Source: CAD feature listing. Evaluate the final solid. Frame: model axes, mm. Face numbers are marked on the shaded views. A direction names the side the tool comes from. Give positions to 0.01 mm unless a question says otherwise; leave off trailing zeros. Loops run counter-clockwise (first coordinate to the right, second up) from the corner with the lowest first, then second, coordinate; pieces in that order, holes last. Notation, with made-up numbers: M -31,79 L -15,79 A29 ccw -15,112 Z; hole C 41.5,0 d2. An arc over 180 degrees is marked long. Answer in a Markdown table with one row per item.
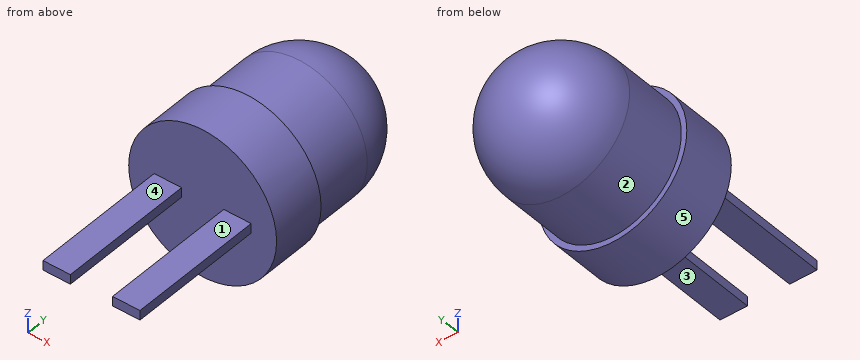
```python
from build123d import *

# Parameters (mm, degrees)
SKETCH2_W                = 1
SKETCH2_H                = 0.35
BOSS_EXTRUDE1_DEPTH      = 5
BOSS_EXTRUDE1_DEPTH_BACK = 5


with BuildPart() as part:
    # Sketch1 → Revolve1 (revolve)
    with BuildSketch(Plane.XY):
        with BuildLine():
            Line((0, 0), (0, 6.825))
            ThreePointArc((0, 6.825), (1.767766953, 6.092766953), (2.5, 4.325))
            Line((2.5, 4.325), (2.5, 2))
            Line((2.5, 2), (2.7, 2))
            Line((2.7, 2), (2.7, 0))
            Line((2.7, 0), (0, 0))
        make_face()
    revolve(axis=Axis((0, 0, 0), (0, 1, 0)))

    # Sketch2 → Boss-Extrude1 (add, two sides)
    with BuildSketch(Plane.XZ) as boss_extrude1_sk:
        with Locations((1.27, 0)):
            Rectangle(SKETCH2_W, SKETCH2_H)
        with Locations((-1.27, 0)):
            Rectangle(SKETCH2_W, SKETCH2_H)
    extrude(amount=BOSS_EXTRUDE1_DEPTH)
    extrude(boss_extrude1_sk.sketch, amount=-BOSS_EXTRUDE1_DEPTH_BACK)


solid = part.part
```
1) Pin query (flat end, axial travel): pin 1 Ø1.1 at (x, y) = (1, -3) entering from -Z (3 decimals); pin 2 Ø1.5 at (y, z) = (2.5, 0) entering from -X; pin 3 Ø1 at (x, y) = (1.5, 0) entering from -Z. Return the tip coordinate at first contact, or that it passes through.
Reply:
| item | result |
|---|---|
| pin 1 | stops at z = -0.175 |
| pin 2 | stops at x = -2.7 |
| pin 3 | stops at z = -2.51 |
2) Material intervals for L1, parallel to Y at x = -2.4, z = -1.1; L2, parallel to Z at x = 1.8, y = 2.75; L3, parallel to X at y = 2.75, z = -1.05, sorted ascending.
Reply:
| item | result |
|---|---|
| L1 | y = 0 to 2 |
| L2 | z = -1.73 to 1.73 |
| L3 | x = -2.27 to 2.27 |
3) Section C-C, the plane x = 0. Return loops of the section in (y, z) (3 decimals).
Reply:
| item | result |
|---|---|
| outline | M 0,-2.7 L 2,-2.7 L 2,-2.5 L 4.325,-2.5 A2.5 ccw 4.325,2.5 L 2,2.5 L 2,2.7 L 0,2.7 Z |
4) Section D-D, the plane y = 2.75. Return loops of the section in (x, z), then the cut area to 3 significant figures.
Reply:
| item | result |
|---|---|
| outline | C 0,0 d5 |
| area | 19.6 mm² |
5) Pull-direction query (X, two-part tool) for the marked faces 4 and 5; classes: released by +X, released by -X, zero draft, split by the parting line, or undercut.
Reply:
| item | result |
|---|---|
| face 4 | zero draft |
| face 5 | split by the parting line |
6) Set-up query: the marked faces 1, 2 and 3. Return all of +Z, -Z, +X, -X, +Y, -Y with unobstructed straight access to the full face (end or side cutting, diameter ignored); none if empty.
Reply:
| item | result |
|---|---|
| face 1 | +Z, +X, -X, -Y |
| face 2 | +Y |
| face 3 | -Z, +X, -X, -Y |
7) Section B-B, the plane z = 0. Return loops of the section in (x, y) (3 decimals), then the cut area to 3 significant figures.
Reply:
| item | result |
|---|---|
| outline | M -2.7,0 L -1.77,0 L -1.77,-5 L -0.77,-5 L -0.77,0 L 0.77,0 L 0.77,-5 L 1.77,-5 L 1.77,0 L 2.7,0 L 2.7,2 L 2.5,2 L 2.5,4.325 A2.5 ccw -2.5,4.325 L -2.5,2 L -2.7,2 Z |
| area | 42.2 mm² |
8) Section A-A, the plane y = -0.5. Return loops of the section in (x, z) (3 decimals).
Reply:
| item | result |
|---|---|
| outline | M -1.77,-0.175 L -0.77,-0.175 L -0.77,0.175 L -1.77,0.175 Z; M 0.77,-0.175 L 1.77,-0.175 L 1.77,0.175 L 0.77,0.175 Z |
